from build123d import *

# Parameters (mm, degrees)
F1_DEPTH = 190.5
F2_R     = 3.175
F3_DEPTH = 25.4
F5_DEPTH = 68.1482
F6_R     = 6.35
F7_DEPTH = 21.9964


with BuildPart() as f1:
    # F0 (on Front) → F1 (new body)
    with BuildSketch(Plane.XZ):
        with BuildLine():
            Line((-35.4203, 61.3497592193), (0, 0))
            Line((0, 0), (7.3406, 0))
            Line((7.3406, 0), (210.5406, 0))
            Line((210.5406, 0), (210.5406, 12.7))
            Line((210.5406, 12.7), (12.1031, 12.7))
            ThreePointArc((12.1031, 12.7), (4.9595820343, 8.5754200581), (4.9588859541, 16.8241780337))
            Line((4.9588859541, 16.8241780337), (-24.4217773719, 67.6997592193))
            Line((-24.4217773719, 67.6997592193), (-35.4203, 61.3497592193))
        make_face()
    extrude(amount=F1_DEPTH)

    # F2 (on face) → F3 (cut)
    with BuildSketch(Plane.XY.offset(12.7)):
        with Locations((108.9406, -12.7)):
            Circle(F2_R)
        with Locations((108.9406, -76.2)):
            Circle(F2_R)
        with Locations((159.7406, -12.7)):
            Circle(F2_R)
        with Locations((108.9406, -152.4)):
            Circle(F2_R)
    extrude(amount=-F3_DEPTH, mode=Mode.SUBTRACT)

    # F4 (on face) → F5 (join)
    with BuildSketch(Plane.XY.offset(12.7)):
        with BuildLine():
            ThreePointArc((51.7906, -12.7), (49.9307280605, -8.2098719395), (45.4406, -6.35))
            Line((45.4406, -6.35), (45.4406, -12.7))
            Line((45.4406, -12.7), (51.7906, -12.7))
        make_face()
        with BuildLine():
            Line((45.4406, -12.7), (45.4406, -6.35))
            ThreePointArc((45.4406, -6.35), (40.9504719395, -17.1901280605), (51.7906, -12.7))
            Line((51.7906, -12.7), (45.4406, -12.7))
        make_face()
    extrude(amount=F5_DEPTH)

    # F6 (on face) → F7 (join)
    with BuildSketch(Plane(origin=(11.0047103243, 0, 6.3552234983), x_dir=(0, 1, 0), z_dir=(0.8659691409, 0, 0.5000974375))):
        with Locations((-12.7, 45.4391706143)):
            Circle(F6_R)
    extrude(amount=F7_DEPTH)


solid = f1.part
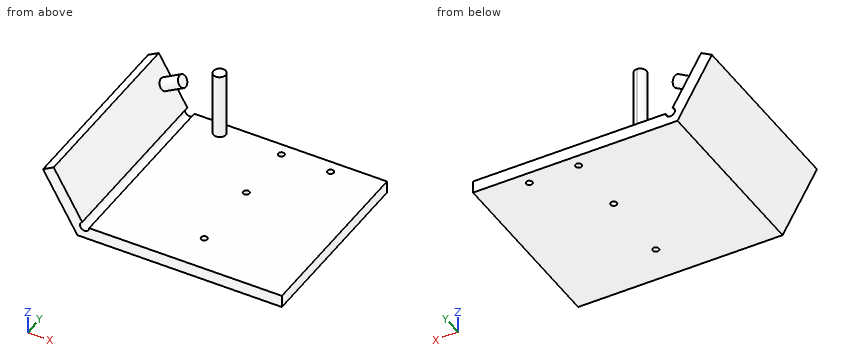
Work out the finished part from the listing and answer in its coordinate system (mm). Round coordinates to 2 decimals unless told otherwise and drop trailing zeros. Loops run counter-clockwise (first coordinate to the right, second up) from the corner with the lowest first, then second, coordinate; pieces in that order, holes last. Notation, with made-up numbers: (74.25, 64.25) - (128.25, 64.25) arc R25 cw to (128.25, 82.25) - close; hole circle Ø11 at (70.25, -34). An arc over 180 degrees is marked (long way). One line per item, written item: value.
Q1. Find section C-C on x = 150.5. Give the vertices of the cut face in (y, z), and give its area (3 significant figures).
Check values:
outline: (-190.5, 0) - (0, 0) - (0, 12.7) - (-190.5, 12.7) - close
area: 2,420 mm2
Q2. Find section B-B on y = -112. Give the vertices of the cut face in (x, z) (1 decimal).
Check values:
outline: (-35.4, 61.3) - (0, 0) - (210.5, 0) - (210.5, 12.7) - (12.1, 12.7) arc R4.8 cw (long way) to (5, 16.8) - (-24.4, 67.7) - close
Q3. Straight lines are drawn through the part: probe 1 along X at (y, z) = (-12, 6); probe 2 along Z at (x, y) = (25, -175); probe 3 along X at (y, z) = (-12, 5). For each, find the intervals that lie inside material, in ascending order.
Check values:
probe 1: -3.46 to 105.84, 112.04 to 156.64, 162.84 to 210.54
probe 2: 0 to 12.7
probe 3: -2.89 to 105.84, 112.04 to 156.64, 162.84 to 210.54
Q4. Find section A-A on y = -76.2. Give the vertices of the cut face in (x, z) (1 decimal), and give its area (3 significant figures).
Check values:
outline: (-35.4, 61.3) - (0, 0) - (105.8, 0) - (105.8, 12.7) - (12.1, 12.7) arc R4.8 cw (long way) to (5, 16.8) - (-24.4, 67.7) - close; (112.1, 0) - (210.5, 0) - (210.5, 12.7) - (112.1, 12.7) - close
area: 3,350 mm2
Q5. Each of these flat-tipped pins is pushed along its axis until it touches: pin 1 Ø7.5 at (x, y) = (108.94, -12.7) entering from +Z; pin 2 Ø12 at (y, z) = (-124.5, 41.5) entering from +X; pin 3 Ø2 at (x, y) = (167, -118) entering from -Z; pin 4 Ø6 at (y, z) = (-60.5, 69) entering from -X. Where does it stop, or does it pass through?
Check values:
pin 1: z = 12.7
pin 2: x = -5.83
pin 3: z = 0
pin 4: x = -27.37
